from build123d import *

# Parameters (mm, degrees)
SKETCH_1_W           = 41
SKETCH_1_H           = 31
SKETCH_1_W_2         = 31
SKETCH_1_H_2         = 21
EXTRUDE_1_DEPTH      = 5
SKETCH_2_W           = 41
SKETCH_2_H           = 31
EXTRUDE_1_2_DEPTH    = 2
CUT_EXTRUDE_START    = -7
SKETCH_3_R           = 1.7
CUT_EXTRUDE_1_DEPTH  = 2
SKETCH_4_R           = 0.7
CUT_EXTRUDE_2_DEPTH  = 27.182054923
FILLET_1_R           = 1
CUT_EXTRUDE_3_DEPTH  = 5
CUT_EXTRUDE_5_DEPTH  = 1
EXTRUDE_START        = 1
EXTRUDE_2_DEPTH      = 1
SKETCH_12_W          = 31
SKETCH_12_H          = 0.5
SKETCH_12_W_2        = 0.5
SKETCH_12_H_2        = 21
CUT_EXTRUDE_9_DEPTH  = 4
EXTRUDE_3_DEPTH      = 1.6
SKETCH_18_W          = 31
SKETCH_18_H          = 0.5
EXTRUDE_4_DEPTH      = 3.6
SKETCH_14_W          = 6.5
SKETCH_14_H          = 6
CUT_EXTRUDE_10_DEPTH = 2
SKETCH_16_R          = 0.9
CUT_EXTRUDE_12_DEPTH = 10
SKETCH_17_W          = 2
SKETCH_17_H          = 1.850967132
CUT_EXTRUDE_13_DEPTH = 2
SKETCH_19_W          = 0.5
SKETCH_19_H          = 21
CUT_EXTRUDE_14_DEPTH = 2
EXTRUDE_5_DEPTH      = 2


with BuildPart() as part:
    # 草图1 → Extrude 1 (new body)
    with BuildSketch(Plane.XY):
        Rectangle(SKETCH_1_W, SKETCH_1_H)
        Rectangle(SKETCH_1_W_2, SKETCH_1_H_2, mode=Mode.SUBTRACT)
    extrude(amount=EXTRUDE_1_DEPTH)

    # 草图2 → Extrude 1 2 (add)
    with BuildSketch(Plane.XY.offset(5)):
        Rectangle(SKETCH_2_W, SKETCH_2_H)
    extrude(amount=EXTRUDE_1_2_DEPTH)

    # 草图3 → 切除-拉伸1 (cut)
    with BuildSketch(Plane(origin=(0, 0, 0), x_dir=(-1, 0, 0), z_dir=(0, 0, -1)).offset(CUT_EXTRUDE_START)):
        with Locations(Location((17.5, 12.5, 0), (0, 0, 180))):
            Circle(SKETCH_3_R)
        with Locations(Location((-17.5, 12.5, 0), (0, 0, 180))):
            Circle(SKETCH_3_R)
        with Locations(Location((17.5, -12.5, 0), (0, 0, 180))):
            Circle(SKETCH_3_R)
        with Locations(Location((-17.5, -12.5, 0), (0, 0, 180))):
            Circle(SKETCH_3_R)
    extrude(amount=CUT_EXTRUDE_1_DEPTH, mode=Mode.SUBTRACT)

    # 草图4 → 切除-拉伸2 (cut, through all)
    with BuildSketch(Plane.XY.offset(5)):
        with Locations((17.5, 12.5)):
            Circle(SKETCH_4_R)
        with Locations(Location((-17.5, 12.5, 0), (0, 0, 180))):
            Circle(SKETCH_4_R)
        with Locations(Location((17.5, -12.5, 0), (0, 0, 180))):
            Circle(SKETCH_4_R)
        with Locations((-17.5, -12.5)):
            Circle(SKETCH_4_R)
    extrude(amount=-CUT_EXTRUDE_2_DEPTH, mode=Mode.SUBTRACT)

    # 圆角1
    fillet_1_edges = [part.edges().sort_by_distance(p)[0] for p in [
        (20.5, -15.5, 3.5),
        (-20.5, -15.5, 3.5),
        (-20.5, 15.5, 3.5),
        (20.5, 15.5, 3.5),
    ]]
    fillet(fillet_1_edges, radius=FILLET_1_R)

    # 草图5 → 切除-拉伸3 (cut)
    with BuildSketch(Plane(origin=(0, 0, 0), x_dir=(-1, 0, 0), z_dir=(0, 0, -1))):
        Polygon((-15.5, 10.5), (-15.5, 12.5), (-15.5, 13.995698298), (15.5, 13.995698298), (15.5, 12.5), (15.5, 10.5), (17.5, 10.5), (19, 10.5), (19, -10.5), (17.5, -10.5), (15.5, -10.5), (15.5, -12.5), (15.5, -14), (-15.5, -14), (-15.5, -12.5), (-15.5, -10.5), (-17.5, -10.5), (-19, -10.5), (-19, 10.5), (-17.5, 10.5), align=None)
    extrude(amount=-CUT_EXTRUDE_3_DEPTH, mode=Mode.SUBTRACT)

    # 草图7 → 切除-拉伸5 (cut)
    with BuildSketch(Plane(origin=(0, 0, 5), x_dir=(-1, 0, 0), z_dir=(0, 0, -1))):
        Polygon((-15.5, 13.995698298), (15.5, 13.995698298), (15.5, 10.5), (19, 10.5), (19, -10.5), (15.5, -10.5), (15.5, -14), (-15.5, -14), (-15.5, -10.5), (-19, -10.5), (-19, -8.940076883), (-19, 8.940076883), (-19, 10.5), (-15.5, 10.5), align=None)
        with BuildLine():
            Line((-8, 8.940076883), (-8, -8.940076883))
            Line((-8, -8.940076883), (-3.073544042, -8.940076883))
            ThreePointArc((-3.073544042, -8.940076883), (12.960986832, -7.047035902), (11.02046595, 8.981818182))
            Line((11.02046595, 8.981818182), (9.242799076, 8.981818182))
            ThreePointArc((9.242799076, 8.981818182), (4.041122306, -10.399918699), (-1.31366402, 8.940076883))
            Line((-1.31366402, 8.940076883), (-4.642515442, 8.940076883))
            Line((-4.642515442, 8.940076883), (-8, 8.940076883))
        make_face(mode=Mode.SUBTRACT)
    extrude(amount=-CUT_EXTRUDE_5_DEPTH, mode=Mode.SUBTRACT)

    # 草图9 → 凸台-拉伸2 (add)
    with BuildSketch(Plane(origin=(0, 0, 5), x_dir=(-1, 0, 0), z_dir=(0, 0, -1)).offset(EXTRUDE_START)):
        with BuildLine():
            Line((-8, 8.940076883), (-1.31366402, 8.940076883))
            ThreePointArc((-1.31366402, 8.940076883), (4, -10.4), (9.31366402, 8.940076883))
            Line((9.31366402, 8.940076883), (11.073544042, 8.940076883))
            ThreePointArc((11.073544042, 8.940076883), (12.940076883, -7.073544042), (-3.073544042, -8.940076883))
            Line((-3.073544042, -8.940076883), (-8, -8.940076883))
            Line((-8, -8.940076883), (-8, 8.940076883))
        make_face()
    extrude(amount=-EXTRUDE_2_DEPTH)

    # 草图12 → 切除-拉伸9 (cut)
    with BuildSketch(Plane(origin=(0, 0, 0), x_dir=(-1, 0, 0), z_dir=(0, 0, -1))):
        with Locations((0, -14.25)):
            Rectangle(SKETCH_12_W, SKETCH_12_H)
        with Locations((0, 14.245698298)):
            Rectangle(SKETCH_12_W, SKETCH_12_H)
        with Locations((-19.25, 0)):
            Rectangle(SKETCH_12_W_2, SKETCH_12_H_2)
        with Locations((19.25, 0)):
            Rectangle(SKETCH_12_W_2, SKETCH_12_H_2)
    extrude(amount=-CUT_EXTRUDE_9_DEPTH, mode=Mode.SUBTRACT)

    # 草图13 → 凸台-拉伸3 (add)
    with BuildSketch(Plane(origin=(0, 0, 0), x_dir=(-1, 0, 0), z_dir=(0, 0, -1))):
        with BuildLine():
            Line((-19.5, 15.5), (19.5, 15.5))
            ThreePointArc((19.5, 15.5), (20.207106781, 15.207106781), (20.5, 14.5))
            Line((20.5, 14.5), (20.5, -14.5))
            ThreePointArc((20.5, -14.5), (20.207106781, -15.207106781), (19.5, -15.5))
            Line((19.5, -15.5), (-19.5, -15.5))
            ThreePointArc((-19.5, -15.5), (-20.207106781, -15.207106781), (-20.5, -14.5))
            Line((-20.5, -14.5), (-20.5, 14.5))
            ThreePointArc((-20.5, 14.5), (-20.207106781, 15.207106781), (-19.5, 15.5))
        make_face()
        with BuildLine():
            Line((-19.5, 13.495698298), (-19.5, -13.5))
            ThreePointArc((-19.5, -13.5), (-19.207106781, -14.207106781), (-18.5, -14.5))
            Line((-18.5, -14.5), (18.5, -14.5))
            ThreePointArc((18.5, -14.5), (19.207106781, -14.207106781), (19.5, -13.5))
            Line((19.5, -13.5), (19.5, 13.495698298))
            ThreePointArc((19.5, 13.495698298), (19.207106781, 14.20280508), (18.5, 14.495698298))
            Line((18.5, 14.495698298), (-18.5, 14.495698298))
            ThreePointArc((-18.5, 14.495698298), (-19.207106781, 14.20280508), (-19.5, 13.495698298))
        make_face(mode=Mode.SUBTRACT)
    extrude(amount=EXTRUDE_3_DEPTH)

    # 草图18 → 凸台-拉伸4 (add)
    with BuildSketch(Plane(origin=(0, 0, 4), x_dir=(-1, 0, 0), z_dir=(0, 0, -1))):
        with Locations((0, 14.245698298)):
            Rectangle(SKETCH_18_W, SKETCH_18_H)
    extrude(amount=EXTRUDE_4_DEPTH)

    # 草图14 → 切除-拉伸10 (cut)
    with BuildSketch(Plane(origin=(0, 15.5, 0), x_dir=(1, 0, 0), z_dir=(0, 1, 0))):
        Polygon((-1, 1.6), (-1, -0.4), (-3, -0.4), (-3, -3), (4, -3), (4, -0.4), (1.5, -0.4), (1.5, 1.6), align=None)
        with Locations((-9.65, -1)):
            Rectangle(SKETCH_14_W, SKETCH_14_H)
    extrude(amount=-CUT_EXTRUDE_10_DEPTH, mode=Mode.SUBTRACT)

    # 草图16 → 切除-拉伸12 (cut)
    with BuildSketch(Plane(origin=(0, 0, 6), x_dir=(-1, 0, 0), z_dir=(0, 0, -1))):
        with Locations((4, 3)):
            Circle(SKETCH_16_R)
        with Locations((7, 0)):
            Circle(SKETCH_16_R)
        with Locations((4, -3)):
            Circle(SKETCH_16_R)
        with Locations((1, 0)):
            Circle(SKETCH_16_R)
        with Locations((4, 6)):
            Circle(SKETCH_16_R)
        with Locations((4, 9)):
            Circle(SKETCH_16_R)
        with Locations((8.5, 7.794228634)):
            Circle(SKETCH_16_R)
        with Locations((11.794228634, 4.5)):
            Circle(SKETCH_16_R)
        with Locations((13, 0)):
            Circle(SKETCH_16_R)
        with Locations((11.794228634, -4.5)):
            Circle(SKETCH_16_R)
        with Locations((8.5, -7.794228634)):
            Circle(SKETCH_16_R)
        with Locations((4, -9)):
            Circle(SKETCH_16_R)
        with Locations((-0.5, -7.794228634)):
            Circle(SKETCH_16_R)
        with Locations((-3.794228634, -4.5)):
            Circle(SKETCH_16_R)
        with Locations((-5, 0)):
            Circle(SKETCH_16_R)
        with Locations((-3.794228634, 4.5)):
            Circle(SKETCH_16_R)
        with Locations((-0.5, 7.794228634)):
            Circle(SKETCH_16_R)
        with Locations((8.242640687, 4.242640687)):
            Circle(SKETCH_16_R)
        with Locations((10, 0)):
            Circle(SKETCH_16_R)
        with Locations((8.242640687, -4.242640687)):
            Circle(SKETCH_16_R)
        with Locations((4, -6)):
            Circle(SKETCH_16_R)
        with Locations((-0.242640687, -4.242640687)):
            Circle(SKETCH_16_R)
        with Locations((-2, 0)):
            Circle(SKETCH_16_R)
        with Locations((-0.242640687, 4.242640687)):
            Circle(SKETCH_16_R)
    extrude(amount=-CUT_EXTRUDE_12_DEPTH, mode=Mode.SUBTRACT)

    # 草图17 → 切除-拉伸13 (cut)
    with BuildSketch(Plane(origin=(0, 0, 4), x_dir=(-1, 0, 0), z_dir=(0, 0, -1))):
        with Locations((-2.31366402, 8.014593317)):
            Rectangle(SKETCH_17_W, SKETCH_17_H)
        Polygon((9.242799076, 8.981818182), (11.242799076, 8.981818182), (10.275574211, 8.014593317), align=None)
    extrude(amount=-CUT_EXTRUDE_13_DEPTH, mode=Mode.SUBTRACT)

    # 草图19 → 切除-拉伸14 (cut)
    with BuildSketch(Plane(origin=(0, 0, 4), x_dir=(-1, 0, 0), z_dir=(0, 0, -1))):
        with Locations((-19.25, 0)):
            Rectangle(SKETCH_19_W, SKETCH_19_H)
    extrude(amount=-CUT_EXTRUDE_14_DEPTH, mode=Mode.SUBTRACT)

    # 草图20 → 凸台-拉伸5 (add)
    with BuildSketch(Plane(origin=(0, 0, 4), x_dir=(-1, 0, 0), z_dir=(0, 0, -1))):
        with BuildLine():
            ThreePointArc((8, -10.675204916), (4, -11.4), (0, -10.675204916))
            Line((0, -10.675204916), (0, -14))
            Line((0, -14), (4, -14))
            Line((4, -14), (8, -14))
            Line((8, -14), (8, -10.675204916))
        make_face()
        with BuildLine():
            Line((19, -4), (19, 0))
            Line((19, 0), (19, 4))
            Line((19, 4), (14.675204916, 4))
            ThreePointArc((14.675204916, 4), (15.217337831, 2.032567829), (15.4, 0))
            ThreePointArc((15.4, 0), (15.217337831, -2.032567829), (14.675204916, -4))
            Line((14.675204916, -4), (19, -4))
        make_face()
    extrude(amount=-EXTRUDE_5_DEPTH)


solid = part.part
Could you check a few things on this model? Use its own coordinates, in mm. A direction names the side the tool comes from. Give positions to 0.01 mm unless a question says otherwise; leave off trailing zeros. Loops run counter-clockwise (first coordinate to the right, second up) from the corner with the lowest first, then second, coordinate; pieces in that order, holes last. Notation, with made-up numbers: (-27, -39) -> (12, -39) arc R14 cw to (12, -16) -> close; hole circle Ø6 at (-36.5, -10.75). An arc over 180 degrees is marked (long way). Return JSON: item names as keys, results as strings.
Item 1: We'd pull the mould along X, two halves only. Please class faces 1 (the cylindrical face through (20.215, 15.199, 2.76)), 2 (the cylindrical face through (0.438, 3.364, 6.493)): +X half, -X half, draft (parallel to the pull), parting line (faces both ways), or undercut.
Geometry results:
{"face 1": "+X half", "face 2": "undercut"}
Item 2: If we section it at A-A on y = 12.5: List the corners of the cut face in (x, z) for me, plus the area to 3 significant figures.
Geometry results:
{"outline": "(-20.5, -1.6) -> (-19.5, -1.6) -> (-19.5, 0) -> (-18.2, 0) -> (-18.2, 5) -> (-19.2, 5) -> (-19.2, 7) -> (-20.5, 7) -> close; (-16.8, 0) -> (-15.5, 0) -> (-15.5, 6) -> (15.5, 6) -> (15.5, 0) -> (16.8, 0) -> (16.8, 5) -> (15.8, 5) -> (15.8, 7) -> (-15.8, 7) -> (-15.8, 5) -> (-16.8, 5) -> close; (18.2, 0) -> (19.5, 0) -> (19.5, -1.6) -> (20.5, -1.6) -> (20.5, 7) -> (19.2, 7) -> (19.2, 5) -> (18.2, 5) -> close", "area": "76.6 mm²"}
Item 3: If we section it at C-C on y = -1.5: List the corners of the cut face in (x, z) for me, plus the area to 3 significant figures.
Geometry results:
{"outline": "(-20.5, -1.6) -> (-19.5, -1.6) -> (-19.5, 4) -> (-14.29, 4) -> (-14.29, 6) -> (6.29, 6) -> (6.29, 4) -> (8, 4) -> (8, 6) -> (19.5, 6) -> (19.5, -1.6) -> (20.5, -1.6) -> (20.5, 7) -> (-20.5, 7) -> close", "area": "70.0 mm²"}
Item 4: Which directions (+Z, -Z, +X, -X, +Y, -Y) give clear straight access to the entire face, cutting with the end or side of a thin tool? Please do faces 3 (the cylindrical face through (-3.805, -6.879, 6.493)), 4 (the flat face through (-12, -14, 5)), 5 (the cylindrical face through (19.07, 13.15, 6.01)), 6 (the flat face through (-2, 15, 0.4)).
Geometry results:
{"face 3": "+Z, -Z", "face 4": "-Z", "face 5": "+Z", "face 6": "+Y"}
Item 5: If we section it at B-B on x = 0.5: Count the separate pieces of the cut face and the enclosed holes in it, plus the area to 3 significant figures.
Geometry results:
{"separate pieces": "5", "enclosed holes": "0", "area": "39.3 mm²"}
Item 6: I need wall thicknesses on L1, parallel to Y at x = 17.5, z = 5.8; L2, parallel to Y at x = 17.5, z = 6.55; L3, parallel to X at y = 12, z = 0.25. Which ranges of each line are inside material? Lowest first, please. Write a range as from..to.
Geometry results:
{"L1": "y = -15.5..-14.2, -10.8..-10.5, 10.5..10.8, 14.2..15.5", "L2": "y = -15.5..-14.2, -10.8..10.8, 14.2..15.5", "L3": "x = -20.5..-17.99, -17.01..-15.5, 15.5..17.01, 17.99..20.5"}
Item 7: I'm going to push flat-ended pins straight in: pin 1 (5 mm diameter, centred on x = 7.5, y = -9.5, fed in from -Z); pin 2 (2.5 mm diameter, centred on x = 0.24, y = -4.24, fed in from -Z). Where does each tip first touch, or does it pass through?
Geometry results:
{"pin 1": "stops at z = 4", "pin 2": "stops at z = 6"}
